The model under review builds one solid part; all positions refer to its coordinate system, in mm. Face numbers are marked on the shaded views. A direction names the side the tool comes from. Coordinates: 2 decimals unless noted, no trailing zeros. Loops run counter-clockwise (first coordinate to the right, second up) from the corner with the lowest first, then second, coordinate; pieces in that order, holes last. Notation, with made-up numbers: (33, 49.25) - (64, 49.25) arc R14 ccw to (64, 58.25) - close; hole circle Ø9 at (-24, 65). An arc over 180 degrees is marked (long way). Use a Markdown table: item, result. Add a question column.
1) Add section C-C, the plane x = -20. Give the boundary of the cut face in (y, z) (3 decimals), and give its area (3 significant figures).
2) Add section D-D, the plane x = 36.5. Give the boundary of the cut face in (y, z) (3 decimals).
3) Add section B-B, the plane z = 7.25. Give the boundary of the cut face in (x, y), and give its area (3 significant figures).
4) Clearance check with flat-ended pins moving along their axes: pin 1 (8 mm diameter, centred on x = 0, z = 5.5, fed in from -Y); pin 2 (2 mm diameter, centred on x = 43, y = 3.5, fed in from +Z); pin 3 (2.5 mm diameter, centred on x = 59, y = -2, fed in from +Z) (3 decimals). State where each tip first meets the part, or that it passes through.
5) Add section A-A, the plane x = 0. Give the boundary of the cut face in (y, z) (3 decimals), and give its area (3 significant figures).
6) The part is to be moulded in two halves that separate along X. For the marked faces 1, 2, 3 and 4, say which applies: pulls with the +X half, pulls with the -X half, needs draft (parallel to the pull), parting line crosses it, or undercut.
7) To check wall thickness, follow L1, parallel to X at y = 59.25, z = 22.05; L2, parallel to Z at x = -21, y = -41; L3, parallel to Y at x = 41.5, z = 1. State the ranges of each line that lie inside material, in increasing order. Write a range as [from, to].
8) For the marked faces 5 and 6, list the 3-axis set-ups (+Z, -Z, +X, -X, +Y, -Y) from which the entire face can be reached by the end or side of a thin tool; tool diameter is ignored.
```python
from build123d import *

# Parameters (mm, degrees)
SKETCH1_R               = 55
BOSS_EXTRUDE1_DEPTH     = 22.825
CUT_EXTRUDE1_REACH      = 152.987
CUT_EXTRUDE1_END_RADIUS = 55
SKETCH3_W               = 5
SKETCH3_H               = 15
BOSS_EXTRUDE2_START     = 4
BOSS_EXTRUDE2_DEPTH     = 4
CUT_EXTRUDE2_REACH      = 107.302
SKETCH6_R               = 1.1
CUT_EXTRUDE3_REACH      = 107.302
SKETCH7_R               = 1.6
CUT_EXTRUDE4_START      = -26.825
SKETCH7_3_R             = 1.6
CUT_EXTRUDE4_DEPTH      = 3


with BuildPart() as part:
    # Sketch1 → Boss-Extrude1 (new body)
    with BuildSketch(Plane.XY):
        with BuildLine():
            Line((-63, 80), (63, 80))
            Line((63, 80), (63, 0))
            ThreePointArc((63, 0), (0, -63), (-63, 0))
            Line((-63, 0), (-63, 80))
        make_face()
        with Locations(Location((0, 0, 0), (0, 0, 90))):
            Circle(SKETCH1_R, mode=Mode.SUBTRACT)
    extrude(amount=BOSS_EXTRUDE1_DEPTH)

    # Cut-Extrude1: up to this cylinder (the profile starts outside it)
    cut_extrude1_end = Plane(origin=(0, 0, 11.4125), z_dir=(0, 0, -1)) * Cylinder(CUT_EXTRUDE1_END_RADIUS, 434.799, mode=Mode.PRIVATE)
    # Sketch3 → Cut-Extrude1 (cut, up to the surface)
    with BuildSketch(Plane(origin=(63, 0, 0), x_dir=(0, 0, -1), z_dir=(1, 0, 0)), mode=Mode.PRIVATE) as cut_extrude1_sk1:
        with Locations((-2.5, 0)):
            Rectangle(SKETCH3_W, SKETCH3_H)
    cut_extrude1_tool1 = extrude(cut_extrude1_sk1.sketch, amount=-CUT_EXTRUDE1_REACH, mode=Mode.PRIVATE) - cut_extrude1_end
    add(cut_extrude1_tool1.solids().sort_by_distance((63, 0, 2.5))[0], mode=Mode.SUBTRACT)
    # Sketch3 → Cut-Extrude1 (cut, up to the surface)
    with BuildSketch(Plane(origin=(63, 0, 0), x_dir=(0, 0, -1), z_dir=(1, 0, 0)), mode=Mode.PRIVATE) as cut_extrude1_sk2:
        with Locations((-20.325, 0)):
            Rectangle(SKETCH3_W, SKETCH3_H)
    cut_extrude1_tool2 = extrude(cut_extrude1_sk2.sketch, amount=-CUT_EXTRUDE1_REACH, mode=Mode.PRIVATE) - cut_extrude1_end
    add(cut_extrude1_tool2.solids().sort_by_distance((63, 0, 20.325))[0], mode=Mode.SUBTRACT)

    # Sketch4 → Boss-Extrude2 (add)
    with BuildSketch(Plane(origin=(0, 0, 0), x_dir=(-1, 0, 0), z_dir=(0, 0, -1)).offset(BOSS_EXTRUDE2_START)):
        with BuildLine():
            Line((63, 0), (63, 80))
            Line((63, 80), (-63, 80))
            Line((-63, 80), (-63, 0))
            ThreePointArc((-63, 0), (0, -63), (63, 0))
        make_face()
    extrude(amount=-BOSS_EXTRUDE2_DEPTH)

    # Sketch6 → Cut-Extrude2 (cut, up to next)
    with BuildSketch(Plane(origin=(0, 0, -4), x_dir=(-1, 0, 0), z_dir=(0, 0, -1)), mode=Mode.PRIVATE) as cut_extrude2_sk1:
        with Locations((5.75, 0)):
            Circle(SKETCH6_R)
    cut_extrude2_tool1 = extrude(cut_extrude2_sk1.sketch, amount=-CUT_EXTRUDE2_REACH, mode=Mode.PRIVATE) & part.part
    # Sketch6 → Cut-Extrude2 (cut, up to next)
    with BuildSketch(Plane(origin=(0, 0, -4), x_dir=(-1, 0, 0), z_dir=(0, 0, -1)), mode=Mode.PRIVATE) as cut_extrude2_sk2:
        with Locations((-5.75, 0)):
            Circle(SKETCH6_R)
    cut_extrude2_tool2 = extrude(cut_extrude2_sk2.sketch, amount=-CUT_EXTRUDE2_REACH, mode=Mode.PRIVATE) & part.part
    add(cut_extrude2_tool1.solids().sort_by_distance((-5.75, 0, -4))[0], mode=Mode.SUBTRACT)
    add(cut_extrude2_tool2.solids().sort_by_distance((5.75, 0, -4))[0], mode=Mode.SUBTRACT)

    # Sketch7 → Cut-Extrude3 (cut, up to next)
    with BuildSketch(Plane(origin=(0, 0, -4), x_dir=(-1, 0, 0), z_dir=(0, 0, -1)), mode=Mode.PRIVATE) as cut_extrude3_sk1:
        with Locations((-41.896076785, 41.896076785)):
            Circle(SKETCH7_R)
    cut_extrude3_tool1 = extrude(cut_extrude3_sk1.sketch, amount=-CUT_EXTRUDE3_REACH, mode=Mode.PRIVATE) & part.part
    # Sketch7 → Cut-Extrude3 (cut, up to next)
    with BuildSketch(Plane(origin=(0, 0, -4), x_dir=(-1, 0, 0), z_dir=(0, 0, -1)), mode=Mode.PRIVATE) as cut_extrude3_sk2:
        with Locations((-41.896076785, -41.896076785)):
            Circle(SKETCH7_R)
    cut_extrude3_tool2 = extrude(cut_extrude3_sk2.sketch, amount=-CUT_EXTRUDE3_REACH, mode=Mode.PRIVATE) & part.part
    # Sketch7 → Cut-Extrude3 (cut, up to next)
    with BuildSketch(Plane(origin=(0, 0, -4), x_dir=(-1, 0, 0), z_dir=(0, 0, -1)), mode=Mode.PRIVATE) as cut_extrude3_sk3:
        with Locations((41.896076785, -41.896076785)):
            Circle(SKETCH7_R)
    cut_extrude3_tool3 = extrude(cut_extrude3_sk3.sketch, amount=-CUT_EXTRUDE3_REACH, mode=Mode.PRIVATE) & part.part
    # Sketch7 → Cut-Extrude3 (cut, up to next)
    with BuildSketch(Plane(origin=(0, 0, -4), x_dir=(-1, 0, 0), z_dir=(0, 0, -1)), mode=Mode.PRIVATE) as cut_extrude3_sk4:
        with Locations((41.896076785, 41.896076785)):
            Circle(SKETCH7_R)
    cut_extrude3_tool4 = extrude(cut_extrude3_sk4.sketch, amount=-CUT_EXTRUDE3_REACH, mode=Mode.PRIVATE) & part.part
    add(cut_extrude3_tool1.solids().sort_by_distance((41.896077, 41.896077, -4))[0], mode=Mode.SUBTRACT)
    add(cut_extrude3_tool2.solids().sort_by_distance((41.896077, -41.896077, -4))[0], mode=Mode.SUBTRACT)
    add(cut_extrude3_tool3.solids().sort_by_distance((-41.896077, -41.896077, -4))[0], mode=Mode.SUBTRACT)
    add(cut_extrude3_tool4.solids().sort_by_distance((-41.896077, 41.896077, -4))[0], mode=Mode.SUBTRACT)

    # Sketch7<3> → Cut-Extrude4 (cut)
    with BuildSketch(Plane(origin=(0, 0, -4), x_dir=(-1, 0, 0), z_dir=(0, 0, -1)).offset(CUT_EXTRUDE4_START)):
        with Locations(Location((59.25, 0, 0), (0, 0, 180))):
            Circle(SKETCH7_3_R)
        with Locations(Location((0, 59.25, 0), (0, 0, 180))):
            Circle(SKETCH7_3_R)
    extrude(amount=CUT_EXTRUDE4_DEPTH, mode=Mode.SUBTRACT)


solid = part.part
```
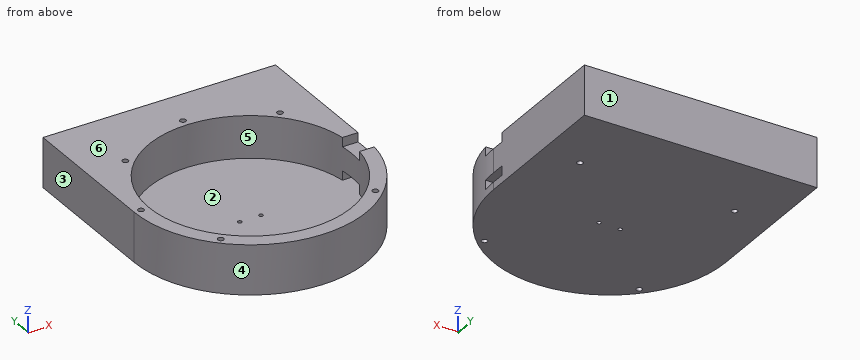
From the geometry:
| question | item | result |
|---|---|---|
| 1 | outline | (-59.741, -4) - (80, -4) - (80, 22.825) - (51.235, 22.825) - (51.235, 0) - (-51.235, 0) - (-51.235, 22.825) - (-59.741, 22.825) - close |
| 1 | area | 1,410 mm^2 |
| 2 | outline | (-51.349, -4) - (80, -4) - (80, 22.825) - (41.143, 22.825) - (41.143, 0) - (-41.143, 0) - (-41.143, 22.825) - (-51.349, 22.825) - close |
| 3 | outline | (-63, 0) arc R63 ccw to (63, 0) - (63, 80) - (-63, 80) - close; hole circle Ø110 at (0, 0); hole circle Ø3.2 at (-41.9, -41.9); hole circle Ø3.2 at (-41.9, 41.9); hole circle Ø3.2 at (41.9, -41.9); hole circle Ø3.2 at (41.9, 41.9) |
| 3 | area | 6,780 mm^2 |
| 4 | pin 1 | stops at y = -63 |
| 4 | pin 2 | stops at z = 0 |
| 4 | pin 3 | stops at z = 17.825 |
| 5 | outline | (-63, -4) - (80, -4) - (80, 22.825) - (60.85, 22.825) - (60.85, 19.825) - (57.65, 19.825) - (57.65, 22.825) - (55, 22.825) - (55, 0) - (-55, 0) - (-55, 22.825) - (-63, 22.825) - close |
| 5 | area | 1,320 mm^2 |
| 6 | face 1 | needs draft |
| 6 | face 2 | undercut |
| 6 | face 3 | pulls with the -X half |
| 6 | face 4 | parting line crosses it |
| 7 | L1 | x = [-63, -1.6], [1.6, 63] |
| 7 | L2 | z = [-4, 0] |
| 7 | L3 | y = [-47.4, -43.45], [-40.35, -36.09], [36.09, 40.35], [43.45, 80] |
| 8 | face 5 | +Z |
| 8 | face 6 | +Z, +X, -X, +Y, -Y |
